Geometry check sheet. Reference: the model listing, model coordinates, mm. Face numbers are marked on the shaded views. A direction names the side the tool comes from. Coordinates: 2 decimals unless noted, no trailing zeros. Loops run counter-clockwise (first coordinate to the right, second up) from the corner with the lowest first, then second, coordinate; pieces in that order, holes last.
from build123d import *

# Parameters (mm, degrees)
F0_R     = 1.75
F0_W     = 20
F0_H     = 15
F1_DEPTH = 9
F2_W     = 12.9252894117
F2_H     = 15.5579744821
F3_DEPTH = 4
F5_DEPTH = 2.5
F7_DEPTH = 25
F8_R     = 1.75
F9_DEPTH = 25
F10_R    = 3


with BuildPart() as f1:
    # F0 (on Top) → F1 (new body)
    with BuildSketch(Plane.XY):
        with BuildLine():
            ThreePointArc((-1.2229712186, -4.3306282914), (2.7153848269, -3.5884098486), (4.5, 0))
            ThreePointArc((4.5, 0), (2.7153848269, 3.5884098486), (-1.2229712186, 4.3306282914))
            ThreePointArc((-1.2229712186, 4.3306282914), (-4.5, 0), (-1.2229712186, -4.3306282914))
        make_face()
        Circle(F0_R, mode=Mode.SUBTRACT)
        with BuildLine():
            ThreePointArc((-1.2229712186, 4.3306282914), (2.7153848269, 3.5884098486), (4.5, 0))
            ThreePointArc((4.5, 0), (2.7153848269, -3.5884098486), (-1.2229712186, -4.3306282914))
            Line((-1.2229712186, -4.3306282914), (10, -7.5))
            Line((10, -7.5), (10, 7.5))
            Line((10, 7.5), (-1.2229712186, 4.3306282914))
        make_face()
        with Locations((20, 0)):
            Rectangle(F0_W, F0_H)
    extrude(amount=F1_DEPTH)

    # F2 (on face) → F3 (cut)
    with BuildSketch(Plane.XY.offset(9)):
        with Locations((-1.4626447058, -0.6304618437)):
            Rectangle(F2_W, F2_H)
    extrude(amount=-F3_DEPTH, mode=Mode.SUBTRACT)

    # F4 (on face) → F5 (cut)
    with BuildSketch(Plane(origin=(0, 0, 0), x_dir=(1, 0, 0), z_dir=(0, 0, -1))):
        Polygon((2.75, -1.5877132403), (2.75, 1.5877132403), (0, 3.1754264805), (-2.75, 1.5877132403), (-2.75, -1.5877132403), (0, -3.1754264805), align=None)
    extrude(amount=-F5_DEPTH, mode=Mode.SUBTRACT)

    # F6 (on face) → F7 (cut)
    with BuildSketch(Plane.XY.offset(9)):
        with BuildLine():
            ThreePointArc((21.4361406616, -4), (23.4760680238, -2.4452916174), (24.25, 0))
            ThreePointArc((24.25, 0), (23.4760680238, 2.4452916174), (21.4361406616, 4))
            Line((21.4361406616, 4), (21.4361406616, -4))
        make_face()
        with BuildLine():
            ThreePointArc((21.4361406616, 4), (23.4760680238, 2.4452916174), (24.25, 0))
            ThreePointArc((24.25, 0), (23.4760680238, -2.4452916174), (21.4361406616, -4))
            Line((21.4361406616, -4), (30, -4))
            Line((30, -4), (30, 4))
            Line((30, 4), (21.4361406616, 4))
        make_face()
        with BuildLine():
            Line((21.4361406616, -4), (21.4361406616, 4))
            ThreePointArc((21.4361406616, 4), (15.75, 0), (21.4361406616, -4))
        make_face()
    extrude(amount=-F7_DEPTH, mode=Mode.SUBTRACT)

    # F8 (on face) → F9 (cut)
    with BuildSketch(Plane.XZ.offset(7.5)):
        with Locations((26, 4.5)):
            Circle(F8_R)
    extrude(amount=-F9_DEPTH, mode=Mode.SUBTRACT)

    # F10
    f10_edges = [f1.edges().sort_by_distance(p)[0] for p in [
        (30, -5.75, 9),
        (30, 5.75, 9),
        (30, -5.75, 0),
        (30, 5.75, 0),
    ]]
    fillet(f10_edges, radius=F10_R)


solid = f1.part
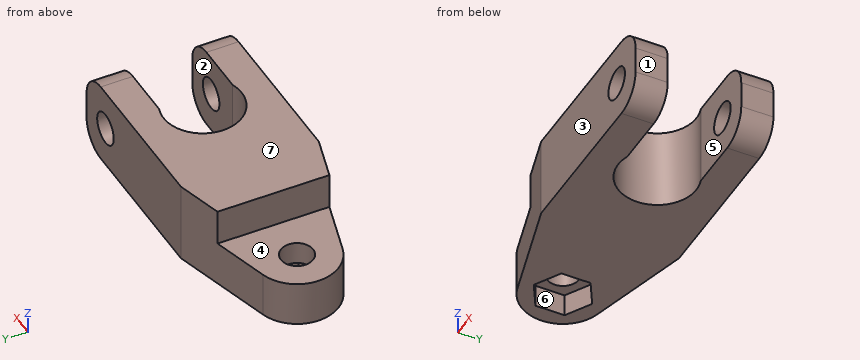
(1) Scan lines: L1, parallel to Y at x = 23, z = 3.25; L2, parallel to Y at x = 20, z = 3.5; L3, parallel to Z at x = 26, y = -5.6. Record each from-to range of solid material in increasing order.
Findings:
L1: y = -7.5 to -4, 4 to 7.5
L2: y = -7.5 to -4.25, 4.25 to 7.5
L3: z = 0 to 2.75, 6.25 to 9
(2) Draft check along Y on the marked faces 1, 2 and 3. Enter one of: +Y half, -Y half, draft (parallel to the pull), parting line (faces both ways), or undercut.
Findings:
face 1: draft
face 2: undercut
face 3: -Y half
(3) Sectioned sample at A-A on z = 4.5. Record the cut outline in (x, y).
Findings:
outline: (-1.22, -4.33) - (10, -7.5) - (24.25, -7.5) - (24.25, -4) - (21.44, -4) arc R4.25 cw (long way) to (21.44, 4) - (24.25, 4) - (24.25, 7.5) - (10, 7.5) - (-1.22, 4.33) arc R4.5 ccw to start; (27.75, -7.5) - (30, -7.5) - (30, -4) - (27.75, -4) - close; (27.75, 4) - (30, 4) - (30, 7.5) - (27.75, 7.5) - close; hole circle Ø3.5 at (0, 0)
(4) Sectioned sample at B-B on x = 26. Record the cut outline in (y, z).
Findings:
outline: (-7.5, 0) - (-4, 0) - (-4, 2.75) - (-7.5, 2.75) - close; (-7.5, 6.25) - (-4, 6.25) - (-4, 9) - (-7.5, 9) - close; (4, 0) - (7.5, 0) - (7.5, 2.75) - (4, 2.75) - close; (4, 6.25) - (7.5, 6.25) - (7.5, 9) - (4, 9) - close
(5) Sectioned sample at C-C on y = 0. Record the cut outline in (x, z).
Findings:
outline: (-4.5, 0) - (-2.75, 0) - (-2.75, 2.5) - (-1.75, 2.5) - (-1.75, 5) - (-4.5, 5) - close; (1.75, 2.5) - (2.75, 2.5) - (2.75, 0) - (15.75, 0) - (15.75, 9) - (5, 9) - (5, 5) - (1.75, 5) - close
(6) Access from +Z, -Z, +X, -X, +Y, -Y to the whole of each face (thin tool, end or side, straight path). Record for the marked faces 4, 5, 6 and 7.
Findings:
face 4: +Z, -X, +Y, -Y
face 5: +Z, -Z, +X
face 6: -Z
face 7: +Z, +X, -X, +Y, -Y
(7) Sectioned sample at D-D on y = -5.25. Record the cut outline in (x, z).
Findings:
outline: (2.03, 0) - (27, 0) arc R3 ccw to (30, 3) - (30, 6) arc R3 ccw to (27, 9) - (5, 9) - (5, 5) - (2.03, 5) - close; hole circle Ø3.5 at (26, 4.5)
(8) Gauge pin test, flat ends, axial feed: pin 1 Ø3 at (x, y) = (0, 0) entering from -Z (3 decimals); pin 2 Ø3 at (y, z) = (-0.5, 1) entering from +X; pin 3 Ø7.5 at (x, y) = (-1.5, 0.5) entering from +Z; pin 4 Ø2 at (y, z) = (3, 7.5) entering from -X. Record the tip position at first contact, or that the pin passes through.
Findings:
pin 1: passes through
pin 2: stops at x = 16.25
pin 3: stops at z = 5
pin 4: stops at x = 5
